The drawing under review shows one solid part. Ordinate dimensions are in mm from its lowest x, y, z. Coordinates: 2 decimals unless noted, no trailing zeros. Write each loop counter-clockwise with the first axis right and the second up, starting at its lowest first coordinate (ties: lowest second). Pieces come first, ordered by that corner, then holes. Notation, with made-up numbers: (20, -35.75) - (78, -35.75) arc R20 ccw to (78, -23.75) - close; hole circle Ø2 at (78, 84.5). An arc over 180 degrees is marked (long way). Use a Markdown table: item, result.
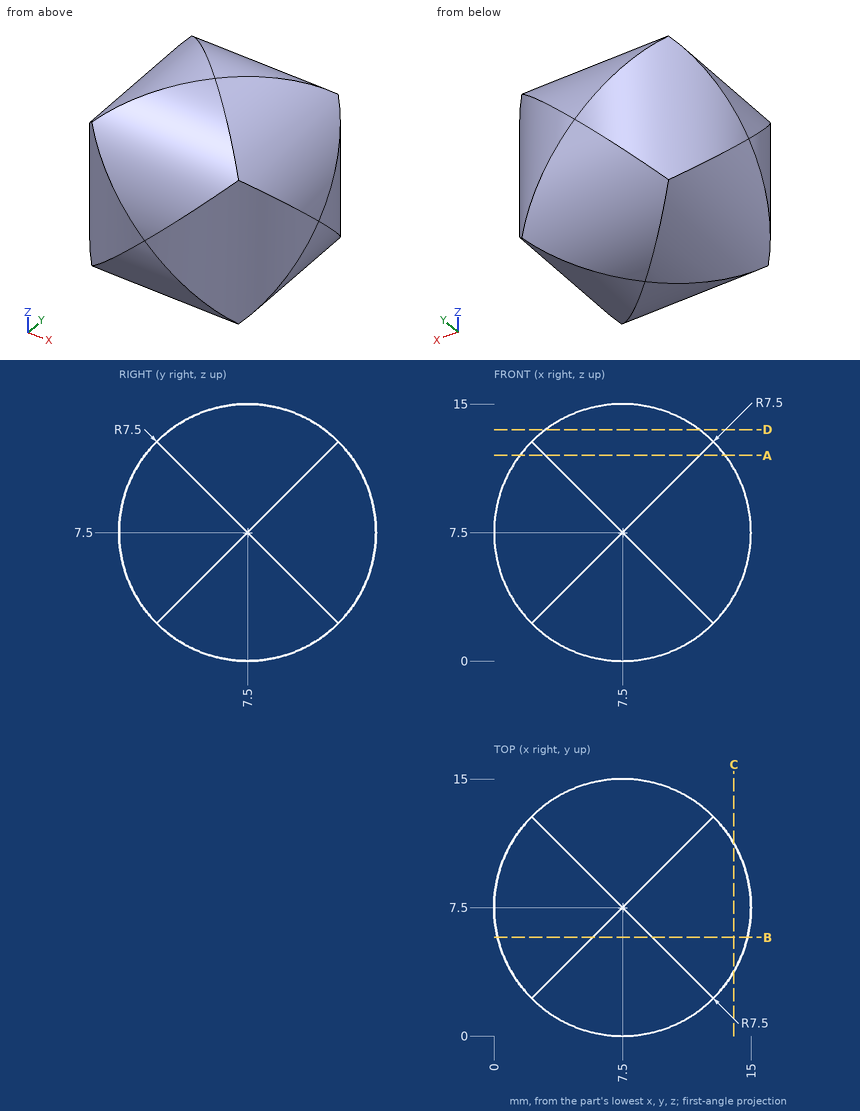
(1) Take a section at B-B on y = 5.75. Write out the cut boundary in (x, z).
Determined:
| item | result |
|---|---|
| outline | (0.21, 5.75) arc R7.5 ccw to (5.75, 0.21) - (9.25, 0.21) arc R7.5 ccw to (14.79, 5.75) - (14.79, 9.25) arc R7.5 ccw to (9.25, 14.79) - (5.75, 14.79) arc R7.5 ccw to (0.21, 9.25) - close |
(2) Take a section at D-D on z = 13.5. Write out the cut boundary in (x, y), and give its area (3 significant figures).
Determined:
| item | result |
|---|---|
| outline | (3, 3) - (12, 3) - (12, 12) - (3, 12) - close |
| area | 81.0 mm2 |
(3) Take a section at C-C on x = 14. Write out the cut boundary in (y, z).
Determined:
| item | result |
|---|---|
| outline | (3.76, 3.76) - (11.24, 3.76) - (11.24, 11.24) - (3.76, 11.24) - close |
(4) For L1, parallel to X at y = 6.25, z = 11.5; L2, parallel to Y at x = 8.5, z = 9.75; L3, parallel to Y at x = 12.5, z = 5.75, list the stretches that pass through material, from the lowest coordinate up. Write a range as from..to.
Determined:
| item | result |
|---|---|
| L1 | 1.16..13.84 |
| L2 | 0.35..14.65 |
| L3 | 1.91..13.09 |
(5) For pin 1 (2 mm diameter, centred on y = 4, z = 9, fed in from -X); pin 2 (1.5 mm diameter, centred on x = 8, y = 4.5, fed in from -Z); pin 3 (1.5 mm diameter, centred on x = 11.5, y = 6, fed in from +Z), all flat-tipped, find the tip position at first contact; note any pin that passes through.
Determined:
| item | result |
|---|---|
| pin 1 | x = 0.43 |
| pin 2 | z = 0.35 |
| pin 3 | z = 14.26 |
(6) Take a section at A-A on z = 12. Write out the cut boundary in (x, y), and give its area (3 significant figures).
Determined:
| item | result |
|---|---|
| outline | (1.5, 3) arc R7.5 ccw to (3, 1.5) - (12, 1.5) arc R7.5 ccw to (13.5, 3) - (13.5, 12) arc R7.5 ccw to (12, 13.5) - (3, 13.5) arc R7.5 ccw to (1.5, 12) - close |
| area | 140 mm2 |
